from build123d import *

# Parameters (mm, degrees)
F1_DEPTH = 24
F2_DEPTH = 8
F3_DEPTH = 16


with BuildPart() as f1:
    # F0 (on Front) → F1 (new body)
    with BuildSketch(Plane.XZ):
        Polygon((0, 15), (0, 0), (42, 0), (42, 15), (28, 15), align=None)
        Polygon((0, 30), (0, 15), (28, 15), (14, 30), align=None)
        Polygon((28, 15), (42, 15), (42, 30), (14, 30), align=None)
    extrude(amount=-F1_DEPTH)

    # F0 (on Front) → F2 (cut)
    with BuildSketch(Plane.XZ):
        Polygon((0, 30), (0, 15), (28, 15), (14, 30), align=None)
        Polygon((28, 15), (42, 15), (42, 30), (14, 30), align=None)
    extrude(amount=-F2_DEPTH, mode=Mode.SUBTRACT)

    # F0 (on Front) → F3 (cut)
    with BuildSketch(Plane.XZ):
        Polygon((28, 15), (42, 15), (42, 30), (14, 30), align=None)
    extrude(amount=-F3_DEPTH, mode=Mode.SUBTRACT)


solid = f1.part
The model under review builds one solid part; all positions refer to its coordinate system, in mm. A direction names the side the tool comes from. Coordinates: 2 decimals unless noted, no trailing zeros. Loops run counter-clockwise (first coordinate to the right, second up) from the corner with the lowest first, then second, coordinate; pieces in that order, holes last. Notation, with made-up numbers: (-31, -15) -> (15, -15) arc R33 ccw to (15, 18) -> close; hole circle Ø7 at (82, -23). An arc over 180 degrees is marked (long way). Use a Markdown table: item, result. Add a question column.
1. Add section C-C on x = 16. Write out the cut boundary in (y, z), plus the area to 3 significant figures.
2. Add section A-A on z = 24. Write out the cut boundary in (x, y).
3. Clearance check with flat-ended pins moving along their axes: pin 1 Ø12 at (x, z) = (8, 23) entering from -Y; pin 2 Ø12 at (x, y) = (24, 9) entering from +Z. State where each tip first meets the part, or that it passes through.
4. To check wall thickness, follow line 1 (Y direction, x = 21, z = 20); line 2 (Z direction, x = 27, y = 3.5); line 3 (Y direction, x = 31, z = 18.25). State the ranges of each line that lie inside material, in increasing order.
5. Add section D-D on x = 20.5. Write out the cut boundary in (y, z).
6. Add section B-B on y = 13.75. Write out the cut boundary in (x, z).
7. Machinability: for faces 1 (the face through (25, 6, 15)), 2 (the face through (0, 14, 15)), 3 (the face through (11, 8, 23)), which of the approach directions +Z, -Z, +X, -X, +Y, -Y give a long, thin tool a straight path to every point of the face, cutting with its end or side? Answer none if there is none.
Returned:
| question | item | result |
|---|---|---|
| 1 | outline | (0, 0) -> (24, 0) -> (24, 30) -> (16, 30) -> (16, 27.86) -> (8, 27.86) -> (8, 15) -> (0, 15) -> close |
| 1 | area | 583 mm² |
| 2 | outline | (0, 8) -> (19.6, 8) -> (19.6, 16) -> (42, 16) -> (42, 24) -> (0, 24) -> close |
| 3 | pin 1 | stops at y = 8 |
| 3 | pin 2 | stops at z = 25.71 |
| 4 | line 1 | y = 8 to 24 |
| 4 | line 2 | z = 0 to 15 |
| 4 | line 3 | y = 16 to 24 |
| 5 | outline | (0, 0) -> (24, 0) -> (24, 30) -> (16, 30) -> (16, 23.04) -> (8, 23.04) -> (8, 15) -> (0, 15) -> close |
| 6 | outline | (0, 0) -> (42, 0) -> (42, 15) -> (28, 15) -> (14, 30) -> (0, 30) -> close |
| 7 | face 1 | +Z, +X, -Y |
| 7 | face 2 | +Z, -Z, -X, +Y, -Y |
| 7 | face 3 | +Z, +X, -X, -Y |
